Geometry: final body of the model. Coordinates: model frame, mm. A direction names the side the tool comes from. Coordinates: 2 decimals unless noted, no trailing zeros. Loops run counter-clockwise (first coordinate to the right, second up) from the corner with the lowest first, then second, coordinate; pieces in that order, holes last. Notation, with made-up numbers: (20, -1) - (55, -1) arc R21 ccw to (55, 28) - close; hole circle Ø5 at (18.25, 57). An arc over 180 degrees is marked (long way). Write each question's results on one line, items separated by ' | '. Start each with the question number.
from build123d import *

# Parameters (mm, degrees)
F1_DEPTH = 240
F3_DEPTH = 240


with BuildPart() as f1:
    # F0 (on Top) → F1 (new body)
    with BuildSketch(Plane.XY):
        with BuildLine():
            Line((800, 0), (0, 0))
            Line((0, 0), (0, -250))
            ThreePointArc((0, -250), (73.223305, -426.776695), (250, -500))
            Line((250, -500), (800, -500))
            Line((800, -500), (800, 0))
        make_face()
    extrude(amount=-F1_DEPTH)

    # F2 (on face) → F3 (join)
    with BuildSketch(Plane(origin=(0, 0, -240), x_dir=(1, 0, 0), z_dir=(0, 0, -1))):
        with BuildLine():
            ThreePointArc((250, 750), (-103.553391, 603.553391), (-250, 250))
            Line((-250, 250), (-250, 0))
            Line((-250, 0), (800, 0))
            Line((800, 0), (800, 750))
            Line((800, 750), (250, 750))
        make_face()
    extrude(amount=F3_DEPTH)


solid = f1.part
1) Section query A-A on y = -216. Output: boundary loops of the cut face in (x, z).
2) Section query C-C on x = 457.5. Output: boundary loops of the cut face in (y, z).
3) Section query D-D on z = -86. Output: boundary loops of the cut face in (x, y), and give its area (3 significant figures).
4) Material intervals for line 1 (X direction, y = -182.5, z = -235.5); line 2 (Z direction, x = 326.5, y = -695.5); line 3 (Y direction, x = 250, z = -101), sorted ascending. Write a range as [from, to].
5) Section query B-B on z = -274. Output: boundary loops of the cut face in (x, y), and give its area (3 significant figures).
6) Pin query (flat end, axial travel): pin 1 Ø2 at (x, z) = (309.5, -130) entering from -Y; pin 2 Ø4 at (x, z) = (-22.5, -420) entering from -Y; pin 3 Ø10 at (x, y) = (253, -516.5) entering from +Z. Return the tip coordinate at first contact, or that it passes through.
7) Access query for faces 1 (the flat face through (521, -500, -118)), 2 (the flat face through (0, -123, -118)), 3 (the cylindrical face through (71.29, -424.82, -118.32)). Directions: +Z, -Z, +X, -X, +Y, -Y. A direction counts if a zero-diameter tool reaches every point of the face in a straight line with its end or side. Return the directions, or none.
Returned:
1) outline: (-250, -480) - (800, -480) - (800, 0) - (0, 0) - (0, -240) - (-250, -240) - close
2) outline: (-750, -480) - (0, -480) - (0, 0) - (-500, 0) - (-500, -240) - (-750, -240) - close
3) outline: (0, -250) arc R250 ccw to (250, -500) - (800, -500) - (800, 0) - (0, 0) - close | area: 387,000 mm²
4) line 1: x = [0, 800] | line 2: z = [-480, -240] | line 3: y = [-500, 0]
5) outline: (-250, -250) arc R500 ccw to (250, -750) - (800, -750) - (800, 0) - (-250, 0) - close | area: 734,000 mm²
6) pin 1: stops at y = -500 | pin 2: stops at y = -670.51 | pin 3: stops at z = -240
7) face 1: +Z, +X, -X, -Y | face 2: +Z, -X, +Y, -Y | face 3: +Z, -X, -Y
